Part model, mm, in its own coordinate system. A direction names the side the tool comes from. Round coordinates to 2 decimals unless told otherwise and drop trailing zeros. Loops run counter-clockwise (first coordinate to the right, second up) from the corner with the lowest first, then second, coordinate; pieces in that order, holes last. Notation, with made-up numbers: (56, -1.75) - (104, -1.75) arc R33 cw to (104, 31.25) - close; hole circle Ø4 at (69.25, -4.75). An arc over 180 degrees is marked (long way). Put each result on its own line as item: value.
from build123d import *

# Parameters (mm, degrees)
SKETCH1_W              = 209.55
SKETCH1_H              = 80.01
BOSS_EXTRUDE1_DEPTH    = 3.175
SKETCH3_R              = 1.89865
CUT_EXTRUDE1_DEPTH     = 113.197510111
SKETCH29_W             = 209.55
SKETCH29_H             = 16.51
CUT_EXTRUDE6_DEPTH     = 113.197510111
BOSS_EXTRUDE6_DEPTH    = 63.5
CUT_EXTRUDE3_DEPTH     = 138.912061642
CUT_EXTRUDE4_DEPTH     = 138.357542769
CUT_EXTRUDE7_REACH     = 139.912
SKETCH30_W             = 50.8
SKETCH30_H             = 18.415
CUT_EXTRUDE9_DEPTH     = 138.912061642
FILLET6_R              = 12.7
FILLET8_R              = 2.54
FILLET9_R              = 3.81
FILLET11_R             = 31.75
CONVERT_SOLID4_START   = -2
CONVERT_SOLID4_DEPTH   = 2
CONVERT_SOLID4_2_DEPTH = 3.175


with BuildPart() as part:
    # Sketch1 → Boss-Extrude1 (new body)
    with BuildSketch(Plane(origin=(0, 0, 0), x_dir=(1, 0, 0), z_dir=(0, 1, 0))):
        Rectangle(SKETCH1_W, SKETCH1_H)
    extrude(amount=BOSS_EXTRUDE1_DEPTH)

    # Sketch3 → Cut-Extrude1 (cut, through all)
    with BuildSketch(Plane(origin=(0, 3.175, 0), x_dir=(1, 0, 0), z_dir=(0, 1, 0))):
        with Locations(Location((36.5125, -14.605, 0), (0, 0, 270))):
            Circle(SKETCH3_R)
        with Locations(Location((14.2875, -14.605, 0), (0, 0, 270))):
            Circle(SKETCH3_R)
        with Locations(Location((-14.2875, -14.605, 0), (0, 0, 270))):
            Circle(SKETCH3_R)
        with Locations(Location((-36.5125, -14.605, 0), (0, 0, 270))):
            Circle(SKETCH3_R)
        with Locations(Location((36.5125, 4.445, 0), (0, 0, 270))):
            Circle(SKETCH3_R)
        with Locations(Location((14.2875, 4.445, 0), (0, 0, 270))):
            Circle(SKETCH3_R)
        with Locations(Location((-14.2875, 4.445, 0), (0, 0, 270))):
            Circle(SKETCH3_R)
        with Locations(Location((-36.5125, 4.445, 0), (0, 0, 270))):
            Circle(SKETCH3_R)
    extrude(amount=-CUT_EXTRUDE1_DEPTH, mode=Mode.SUBTRACT)

    # Sketch29 → Cut-Extrude6 (cut, through all)
    with BuildSketch(Plane(origin=(0, 3.175, 0), x_dir=(1, 0, 0), z_dir=(0, 1, 0))):
        with Locations((0, -31.75)):
            Rectangle(SKETCH29_W, SKETCH29_H)
    extrude(amount=-CUT_EXTRUDE6_DEPTH, mode=Mode.SUBTRACT)

    # Sketch19 → Boss-Extrude6 (add, through all)
    with BuildSketch(Plane(origin=(0, 0, -40.005), x_dir=(-1, 0, 0), z_dir=(0, 0, -1))):
        Polygon((-104.775, 0), (-127.225640303, -22.450640303), (-129.470704333, -20.205576272), (-106.090128061, 3.175), (-104.775, 3.175), align=None)
    boss_extrude6 = extrude(amount=-BOSS_EXTRUDE6_DEPTH)

    # Sketch25 → Cut-Extrude3 (cut, through all)
    with BuildSketch(Plane(origin=(0, 3.175, 0), x_dir=(1, 0, 0), z_dir=(0, 1, 0))):
        with BuildLine():
            Line((144.190128061, 11.508273959), (97.502219088, 5.361694136))
            ThreePointArc((97.502219088, 5.361694136), (75.663289052, -66.631609949), (144.190128061, -35.58250314))
            Line((144.190128061, -35.58250314), (144.190128061, 11.508273959))
        make_face()
    cut_extrude3 = extrude(amount=-CUT_EXTRUDE3_DEPTH, mode=Mode.SUBTRACT)

    # Sketch26 → Cut-Extrude4 (cut, through all)
    with BuildSketch(Plane(origin=(0, 0, 0), x_dir=(0, 0, -1), z_dir=(1, 0, 0))):
        Polygon((40.005, 3.175), (14.379359697, -22.450640303), (40.005, -22.450640303), align=None)
    cut_extrude4 = extrude(amount=CUT_EXTRUDE4_DEPTH, mode=Mode.SUBTRACT)

    # Sketch30 → Cut-Extrude7 (cut, up to next)
    with BuildSketch(Plane(origin=(0, 3.175, 0), x_dir=(1, 0, 0), z_dir=(0, 1, 0)), mode=Mode.PRIVATE) as cut_extrude7_sk1:
        with Locations((0, -14.2875)):
            Rectangle(SKETCH30_W, SKETCH30_H)
    cut_extrude7_tool1 = extrude(cut_extrude7_sk1.sketch, amount=-CUT_EXTRUDE7_REACH, mode=Mode.PRIVATE) & part.part
    add(cut_extrude7_tool1.solids().sort_by_distance((0, 3.175, 14.2875))[0], mode=Mode.SUBTRACT)

    # Mirror9: Boss-Extrude6, Cut-Extrude3, Cut-Extrude4 across plane
    add(boss_extrude6.mirror(Plane(origin=(0, 0, 0), x_dir=(0, 0, 1), z_dir=(1, 0, 0))))
    add(cut_extrude3.mirror(Plane(origin=(0, 0, 0), x_dir=(0, 0, 1), z_dir=(1, 0, 0))), mode=Mode.SUBTRACT)
    add(cut_extrude4.mirror(Plane(origin=(0, 0, 0), x_dir=(0, 0, 1), z_dir=(1, 0, 0))), mode=Mode.SUBTRACT)

    # Sketch32 → Cut-Extrude9 (cut, through all)
    with BuildSketch(Plane(origin=(0, 3.175, 0), x_dir=(1, 0, 0), z_dir=(0, 1, 0))):
        Polygon((-106.090128061, 6.492313801), (-106.090128061, 40.005), (-129.470704333, 16.624423728), (-129.470704333, 9.570425062), align=None)
        Polygon((106.090128061, 6.492313801), (106.090128061, 40.005), (129.470704333, 16.624423728), (129.470704333, 9.570425062), align=None)
    extrude(amount=-CUT_EXTRUDE9_DEPTH, mode=Mode.SUBTRACT)

    # Fillet6
    fillet6_edges = [part.edges().sort_by_distance(p)[0] for p in [
        (-63.403689339, 1.5875, 23.495),
        (63.403689339, 1.5875, 23.495),
    ]]
    fillet(fillet6_edges, radius=FILLET6_R)

    # Fillet8
    fillet8_edges = [part.edges().sort_by_distance(p)[0] for p in [
        (25.4, 1.5875, 5.08),
        (-25.4, 1.5875, 5.08),
    ]]
    fillet(fillet8_edges, radius=FILLET8_R)

    # Fillet9
    fillet9_edges = [part.edges().sort_by_distance(p)[0] for p in [
        (25.4, 1.5875, 23.495),
        (-25.4, 1.5875, 23.495),
    ]]
    fillet(fillet9_edges, radius=FILLET9_R)

    # Fillet11
    # the kernel refuses this fillet: 31.75 mm, written as the material it takes off along each edge
    with BuildSketch(Plane(origin=(-106.090128061, 66.078198255, -6.492313801), x_dir=(0.9786385895506081, 0, 0.20558820744973783), z_dir=(0, -1, 0))) as fillet11_piece_1:
        with BuildLine():
            CenterArc((25.898912909, -31.151224474), FILLET11_R, 101.145067179, 66.990998507)
            Line((-5.172862309, -24.623798888), (-8.280039831, -23.971056329))
            Line((-8.280039831, -23.971056329), (-3.107177522, 0.652742559))
            Line((-3.107177522, 0.652742559), (0.241590205, 3.165795188))
            ThreePointArc((0.241590205, 3.165795188), (8.8784914, 2.506690411), (19.14812824, 3.115122447))
            Line((19.14812824, 3.115122447), (19.761835937, 0))
        make_face()
    extrude(amount=130.296524571, mode=Mode.SUBTRACT)
    with BuildSketch(Plane(origin=(106.090128061, 66.078198255, -6.492313801), x_dir=(-0.9786385895506081, 0, 0.20558820744973783), z_dir=(0, -1, 0))) as fillet11_piece_2:
        with BuildLine():
            CenterArc((25.898912909, 31.151224474), FILLET11_R, 191.863934313, 66.990998507)
            Line((-5.172862309, 24.623798888), (-8.280039831, 23.971056329))
            Line((-8.280039831, 23.971056329), (-3.107177522, -0.652742559))
            Line((-3.107177522, -0.652742559), (0.241590205, -3.165795188))
            ThreePointArc((0.241590205, -3.165795188), (8.8784914, -2.506690411), (19.14812824, -3.115122447))
            Line((19.14812824, -3.115122447), (19.761835937, 0))
        make_face()
    extrude(amount=130.296524571, mode=Mode.SUBTRACT)

    # Convert-Solid4: read off the stored shape, not the designer's step
    # Convert-Solid4 outline → Convert-Solid4 (cut)
    with BuildSketch(Plane(origin=(0, 0, 0), x_dir=(1, 0, 0), z_dir=(0, 1, 0)).offset(CONVERT_SOLID4_START)):
        with BuildLine():
            Line((106.090128061, 31.653593103), (106.090128061, 40.005))
            Line((106.090128061, 40.005), (-106.090128061, 40.005))
            Line((-106.090128061, 40.005), (-106.090128061, 31.653593103))
            ThreePointArc((-106.090128061, 31.653593103), (-105.626557255, 26.247869444), (-104.249381712, 21))
            Line((-104.249381712, 21), (104.249381712, 21))
            ThreePointArc((104.249381712, 21), (105.626557255, 26.247869444), (106.090128061, 31.653593103))
        make_face()
    extrude(amount=CONVERT_SOLID4_DEPTH, mode=Mode.SUBTRACT)

    # Convert-Solid4 2 outline → Convert-Solid4 2 (add)
    with BuildSketch(Plane(origin=(0, 0, 0), x_dir=(1, 0, 0), z_dir=(0, 1, 0))):
        with BuildLine():
            Line((106.090128061, 31.653593103), (106.090128061, 40.005))
            Line((106.090128061, 40.005), (-106.090128061, 40.005))
            Line((-106.090128061, 40.005), (-106.090128061, 31.653593103))
            ThreePointArc((-106.090128061, 31.653593103), (-105.626557255, 26.247869444), (-104.249381712, 21))
            Line((-104.249381712, 21), (104.249381712, 21))
            ThreePointArc((104.249381712, 21), (105.626557255, 26.247869444), (106.090128061, 31.653593103))
        make_face()
    extrude(amount=CONVERT_SOLID4_2_DEPTH)


solid = part.part
1. Band-saw the part on B-B (z = 14.5). List the corners of the cut face in (x, y) (3 decimals).
A:
outline: (-67.382, 0) - (-38.408, 0) - (-38.408, 3.175) - (-67.382, 3.175) - close; (-34.617, 0) - (-25.4, 0) - (-25.4, 3.175) - (-34.617, 3.175) - close; (25.4, 0) - (34.617, 0) - (34.617, 3.175) - (25.4, 3.175) - close; (38.408, 0) - (67.382, 0) - (67.382, 3.175) - (38.408, 3.175) - close
2. Band-saw the part on D-D (x = -93). List the corners of the cut face in (y, z) (3 decimals), plus the area to 3 significant figures.
A:
outline: (0, -40.005) - (3.175, -40.005) - (3.175, -5.966) - (0, -5.966) - close
area: 108 mm²
3. Band-saw the part on A-A (y = 0.8). Give the number of separate pieces and of enclosed holes in the cut face, plus the area to 3 significant figures.
A:
separate pieces: 1
enclosed holes: 6
area: 10,300 mm²
4. Probe line 1 along X through (y, z) = (0.9, 14.5); line 2 along Z through (x, y) = (-35, 2.45) (3 decimals); line 3 along X through (y, z) = (1.4, 13). List the from-to ranges inside material, lowest first. Write a range as [from, to].
A:
line 1: x = [-67.38, -38.41], [-34.62, -25.4], [25.4, 34.62], [38.41, 67.38]
line 2: z = [-40.005, -5.593], [-3.297, 13.457], [15.753, 23.495]
line 3: x = [-68.32, -37.53], [-35.5, -25.4], [25.4, 35.5], [37.53, 68.32]
5. Pin check, flat tips, straight feed: P1, Ø1.6, axis at x = 7, y = 2, coming from the +Z side; P2, Ø3, axis at x = -36.51, z = 14.6, coming from the +Y side; P3, Ø1.5, axis at y = 1, z = -17.5, coming from the +X side; P4, Ø1, axis at y = 2, z = 1.5, coming from the +X side. Stop position of each tip, or through.
A:
P1: stops at z = 5.08
P2: passes through
P3: stops at x = 103.12
P4: stops at x = 80.32
6. Band-saw the part on C-C (x = 1). List the corners of the cut face in (y, z) (3 decimals).
A:
outline: (0, -40.005) - (3.175, -40.005) - (3.175, 5.08) - (0, 5.08) - close
7. Tool access for faces 1 (the cylindrical face through (61.442, 1.61, 21.693)), 2 (the cylindrical face through (26.486, 1.565, 22.349)): list every direction of +Z, -Z, +X, -X, +Y, -Y with a clear straight run to the whole face (end or side of a thin tool).
A:
face 1: +Z, +X, +Y, -Y
face 2: +Z, +Y, -Y
8. Two-plate mould, pull along Z, no slides. Class faces 3 (the cylindrical face through (-38.366, 1.61, -4.857)), 4 (the cylindrical face through (-100.673, 1.61, -13.916)), 5 (the cylindrical face through (-15.443, 1.61, -5.952)), 6 (the flat face through (-1, 0, -16)): pulls with the +Z half, pulls with the -Z half, needs draft (parallel to the pull), parting line crosses it, or undercut.
A:
face 3: undercut
face 4: pulls with the +Z half
face 5: undercut
face 6: needs draft
